```python
from build123d import *

# Parameters (mm, degrees)
SKETCH1_R   = 7.9375
SHAFT_DEPTH = 101.6
HEAD_DEPTH  = 7


with BuildPart() as part:
    # Sketch1 → Shaft (new body)
    with BuildSketch(Plane(origin=(0, 0, 0), x_dir=(1, 0, 0), z_dir=(0, 1, 0))):
        with Locations(Location((0, 0, 0), (0, 0, 270))):
            Circle(SKETCH1_R)
    extrude(amount=-SHAFT_DEPTH)

    # Sketch2 → Head (add)
    with BuildSketch(Plane(origin=(0, 0, 0), x_dir=(1, 0, 0), z_dir=(0, 1, 0))):
        Polygon((11.595031913, -9.533549616), (14.053812112, 5.274817386), (2.458780199, 14.808367002), (-11.595031913, 9.533549616), (-14.053812112, -5.274817386), (-2.458780199, -14.808367002), align=None)
    extrude(amount=HEAD_DEPTH)


solid = part.part
```
The listing builds one solid part. Answer for the finished solid, in the listing's coordinates (mm). A direction names the side the tool comes from. Give positions to 0.01 mm unless a question says otherwise; leave off trailing zeros. Loops run counter-clockwise (first coordinate to the right, second up) from the corner with the lowest first, then second, coordinate; pieces in that order, holes last. Notation, with made-up numbers: M 2.5,6 L 22.5,6 A9 cw 22.5,12 Z; hole C 34,46.5 d1. An arc over 180 degrees is marked long. One line per item, written item: value.
1. Each of these flat-tipped pins is pushed along its axis until it touches: P1, Ø3, axis at x = -7.5, y = -72, coming from the -Z side; P2, Ø3, axis at x = 0, z = -11.5, coming from the -Y side; P3, Ø8, axis at y = -9, z = 9, coming from the -X side. Where does it stop, or does it pass through?
Found:
P1: z = -5.2
P2: y = 0
P3: x = -6.16
2. For faces 1 (the face through (-4.47, 3.451, -12.208)), 2 (the face through (-6, 0, 6)), determine the directions among +Z, -Z, +X, -X, +Y, -Y from which every point of the face is accessible in a straight line to the end or side of a thin tool.
Found:
face 1: -Z, -X, +Y, -Y
face 2: -Y
3. Section A-A on x = 4.75 is taken. Determine the outline of the cut face in (y, z), plus the area to 3 significant figures.
Found:
outline: M -101.6,-6.36 L 0,-6.36 L 0,-12.92 L 7,-12.92 L 7,12.1 L 0,12.1 L 0,6.36 L -101.6,6.36 Z
area: 1,470 mm^2
4. Section B-B on y = -20 is taken. Determine the outline of the cut face in (x, z) (1 decimal).
Found:
outline: C 0,0 d15.9
5. Section C-C on z = 0 is taken. Determine the outline of the cut face in (x, y).
Found:
outline: M -13.18,0 L -7.94,0 L -7.94,-101.6 L 7.94,-101.6 L 7.94,0 L 13.18,0 L 13.18,7 L -13.18,7 Z
6. Section D-D on x = -10.5 is taken. Determine the outline of the cut face in (y, z), plus the area to 3 significant figures.
Found:
outline: M 0,-9.94 L 7,-9.94 L 7,8.2 L 0,8.2 Z
area: 127 mm^2
7. Find the intervals of material crossed by probe 1 along Y at (x, z) = (-10.75, 2.25); probe 2 along X at (y, z) = (-10, 0.25); probe 3 along Z at (x, y) = (5, -55), in increasing order.
Found:
probe 1: 0 to 7
probe 2: -7.93 to 7.93
probe 3: -6.16 to 6.16
